Design review of the part shown in the three views and the two pictorial views. Dimensions are in mm from the part's minimum x, y and z. A direction names the side the tool comes from. Give positions to 0.01 mm unless a question says otherwise; leave off trailing zeros. Loops run counter-clockwise (first coordinate to the right, second up) from the corner with the lowest first, then second, coordinate; pieces in that order, holes last.
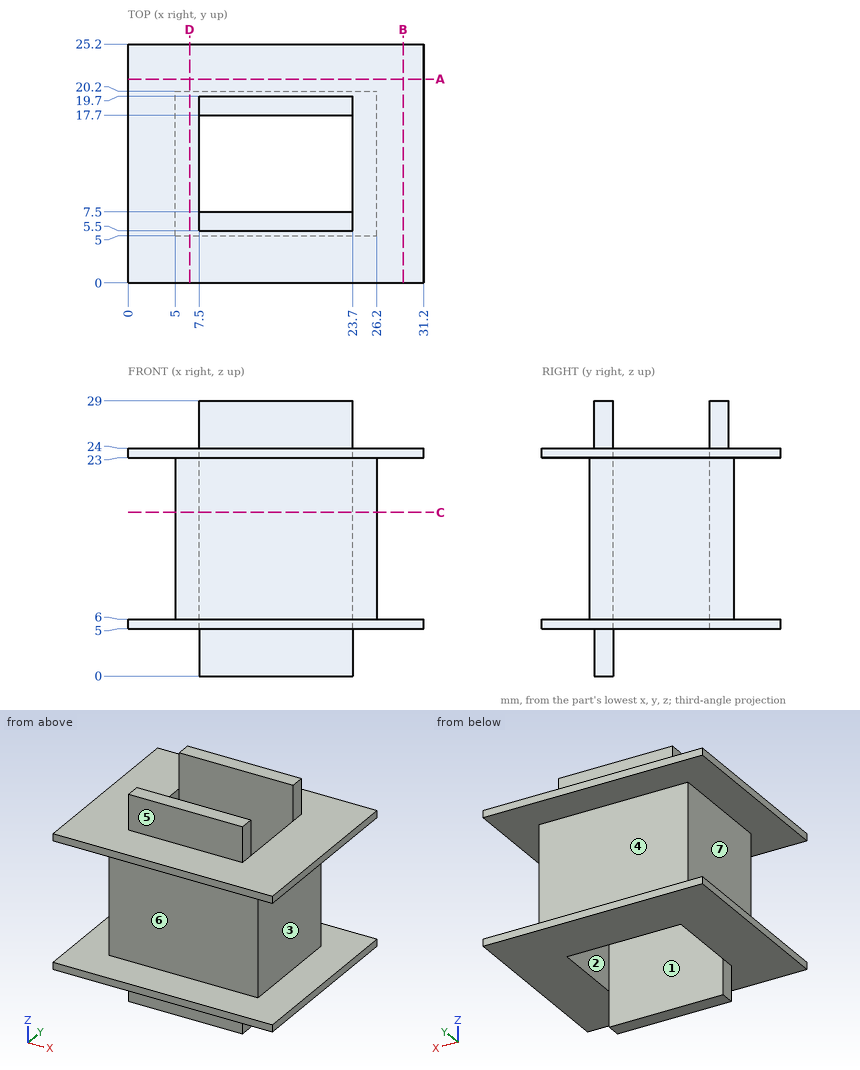
Q1. Tool access review of the marked faces 5, 6 and 7: name each direction out of +Z, -Z, +X, -X, +Y, -Y from which nothing blocks a thin tool from reaching the whole face with its end or side.
Results:
face 5: +Z, +X, -X, -Y
face 6: +X, -X, -Y
face 7: -X, +Y, -Y
Q2. Take a section at A-A (y = 21.5). Give the boundary of the cut face in (x, z).
Results:
outline: (0, 5) - (31.2, 5) - (31.2, 6) - (0, 6) - close; (0, 23) - (31.2, 23) - (31.2, 24) - (0, 24) - close
Q3. Insertion check: pin 1 (7.5 mm diameter, centred on y = 16, z = 16.5, fed in from +X); pin 2 (0.6 mm diameter, centred on y = 18.5, z = 26, fed in from -X); pin 3 (0.6 mm diameter, centred on y = 6.5, z = 27.5, fed in from +X); pin 4 (1.5 mm diameter, centred on x = 4, z = 21.5, fed in from -Y). Each pin has a flat end and moves straight along its axis. Give the tip position at first contact, or say it passes through.
Results:
pin 1: stops at x = 26.2
pin 2: stops at x = 7.5
pin 3: stops at x = 23.7
pin 4: passes through
Q4. Wall thickness on line 1 (Z direction, x = 9, y = 2.25); line 2 (X direction, y = 15, z = 21); line 3 (Y direction, x = 10, z = 13): over which ranges is each line inside the solid? List them lowest first.
Results:
line 1: z = 5 to 6, 23 to 24
line 2: x = 5 to 7.5, 23.7 to 26.2
line 3: y = 5 to 7.5, 17.7 to 20.2
Q5. Draft analysis for pull direction X (two halves, no side actions). For the marked faces 1, 2, 3 and 4, state which applies: pulls with the +X half, pulls with the -X half, needs draft (parallel to the pull), parting line crosses it, or undercut.
Results:
face 1: undercut
face 2: undercut
face 3: pulls with the +X half
face 4: needs draft
Q6. Take a section at C-C (z = 17.25). Give the boundary of the cut face in (x, y).
Results:
outline: (5, 5) - (26.2, 5) - (26.2, 20.2) - (5, 20.2) - close; hole (7.5, 7.5) - (23.7, 7.5) - (23.7, 17.7) - (7.5, 17.7) - close
Q7. Take a section at D-D (x = 6.5). Give the boundary of the cut face in (y, z), plus the area to 3 significant figures.
Results:
outline: (0, 5) - (25.2, 5) - (25.2, 6) - (20.2, 6) - (20.2, 23) - (25.2, 23) - (25.2, 24) - (0, 24) - (0, 23) - (5, 23) - (5, 6) - (0, 6) - close
area: 309 mm2
Q8. Take a section at B-B (x = 29). Give the boundary of the cut face in (y, z), plus the area to 3 significant figures.
Results:
outline: (0, 5) - (25.2, 5) - (25.2, 6) - (0, 6) - close; (0, 23) - (25.2, 23) - (25.2, 24) - (0, 24) - close
area: 50.4 mm2
